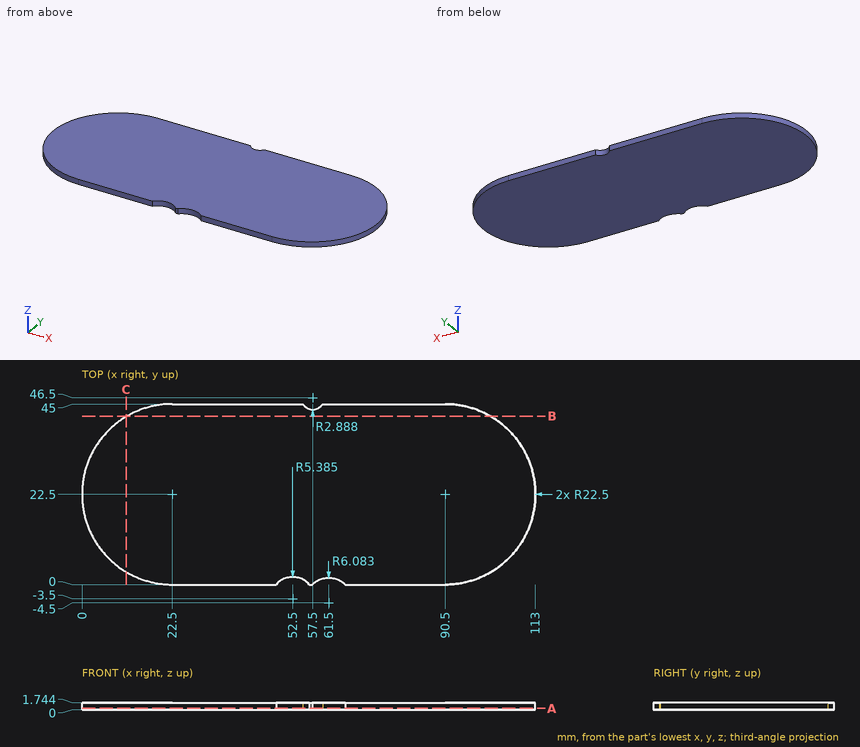
Answer from the drawing. Dimensions are ordinates in mm from the lowest x, y and z of the part. Round coordinates to 2 decimals unless told otherwise and drop trailing zeros. Write each loop counter-clockwise with the first axis right and the second up, starting at its lowest first coordinate (ties: lowest second). Pieces come first, ordered by that corner, then holes. Notation, with made-up numbers: (42.5, 85) - (97.5, 85) arc R15 ccw to (97.5, 94) - close; hole circle Ø1 at (6.25, 32.5). An arc over 180 degrees is marked (long way). Use a Markdown table: item, result.
(1) Straight lines are drawn through the part: line 1 along Y through (x, z) = (22, 0.7) (1 decimal); line 2 along Y through (x, z) = (53, 0.2); line 3 along X through (y, z) = (11.5, 0.6). For each, find the intervals that lie inside material, in ascending order. Write a range as [from, to].
Reported:
| item | result |
|---|---|
| line 1 | [0, 45] |
| line 2 | [1.86, 45] |
| line 3 | [2.87, 110.13] |
(2) The part is cut by section C-C (x = 11). Write down the section's boundary in (y, z).
Reported:
| item | result |
|---|---|
| outline | (3.16, 0) - (41.84, 0) - (41.84, 1.74) - (3.16, 1.74) - close |
(3) The part is cut by section A-A (z = 0.3). Write down the section's boundary in (x, y) (1 decimal), then the cut area to 3 significant figures.
Reported:
| item | result |
|---|---|
| outline | (22.5, 0) - (48.4, 0) arc R5.4 cw to (56.6, 0) - (57.4, 0) arc R6.1 cw to (65.6, 0) - (90.5, 0) arc R22.5 ccw to (90.5, 45) - (60, 45) arc R2.9 cw to (55, 45) - (22.5, 45) arc R22.5 ccw to start |
| area | 4,630 mm2 |
(4) The part is cut by section B-B (y = 42). Write down the section's boundary in (x, z) (1 decimal).
Reported:
| item | result |
|---|---|
| outline | (11.3, 0) - (101.7, 0) - (101.7, 1.7) - (11.3, 1.7) - close |
